```python
from build123d import *

# Parameters (mm, degrees)
SKETCH_1_R           = 7
EXTRUDE_1_DEPTH      = 30
SKETCH_2_W           = 5
SKETCH_2_H           = 5
EXTRUDE_2_DEPTH      = 0.1
EXTRUDE_2_DEPTH_BACK = 20
SKETCH_3_R           = 9
EXTRUDE_3_DEPTH      = 4
SKETCH_4_R           = 80
SKETCH_4_R_2         = 52
EXTRUDE_4_DEPTH      = 10
SKETCH_5_R           = 53
EXTRUDE_5_DEPTH      = 26
SKETCH_7_R           = 55
SKETCH_7_R_2         = 52
EXTRUDE_6_DEPTH      = 7.5
CHAMFER_1_SIZE       = 0.5
SKETCH_8_R           = 5
CUT_EXTRUDE_1_DEPTH  = 31
SKETCH_10_R          = 56
EXTRUDE_7_DEPTH      = 110
SKETCH_11_R          = 56.5
EXTRUDE_8_DEPTH      = 57
CHAMFER_2_SIZE       = 19
EXTRUDE_9_DEPTH      = 100
CUT_EXTRUDE_2_REACH  = 145
SKETCH_13_R          = 3.5
SKETCH_14_W          = 50
SKETCH_14_H          = 50
EXTRUDE_10_DEPTH     = 91
SKETCH_15_R          = 15
EXTRUDE_11_DEPTH     = 58
CHAMFER_3_SIZE       = 1
SKETCH_17_R          = 4
SKETCH_18_R          = 7
EXTRUDE_12_DEPTH     = 4
EXTRUDE_13_DEPTH     = 7
SKETCH_20_R          = 4
CUT_EXTRUDE_3_DEPTH  = 7


with BuildPart() as part:
    # Sketch 1 → Extrude 1 (new body)
    with BuildSketch(Plane.XY):
        Circle(SKETCH_1_R)
    extrude(amount=EXTRUDE_1_DEPTH)

    # Sketch 2 → Extrude 2 (add, two sides)
    with BuildSketch(Plane(origin=(0, 0, 0), x_dir=(-1, 0, 0), z_dir=(0, 0, -1))) as extrude_2_sk:
        with Locations((0, 6.5)):
            Rectangle(SKETCH_2_W, SKETCH_2_H)
    extrude(amount=EXTRUDE_2_DEPTH)
    extrude(extrude_2_sk.sketch, amount=-EXTRUDE_2_DEPTH_BACK)

    # Sketch 3 → Extrude 3 (add)
    with BuildSketch(Plane.XY.offset(30)):
        Circle(SKETCH_3_R)
    extrude(amount=EXTRUDE_3_DEPTH)



with BuildPart() as body_2:
    # Sketch 4 → Extrude 4 (new body)
    with BuildSketch(Plane(origin=(0, 0, 30), x_dir=(-1, 0, 0), z_dir=(0, 0, -1))):
        Circle(SKETCH_4_R)
        Circle(SKETCH_4_R_2, mode=Mode.SUBTRACT)
    extrude(amount=-EXTRUDE_4_DEPTH)


with BuildPart() as part_1:
    add(part.part)

    add(body_2.part)  # Extrude 5 merges body 2
    # Sketch 5 → Extrude 5 (add)
    with BuildSketch(Plane.XY.offset(34)):
        with Locations(Location((0, 0, 0), (0, 0, 180))):  # turned: the seam where the file's is
            Circle(SKETCH_5_R)
    extrude(amount=EXTRUDE_5_DEPTH)

    # Sketch 7 → Extrude 6 (add)
    with BuildSketch(Plane(origin=(0, 0, 34), x_dir=(-1, 0, 0), z_dir=(0, 0, -1))):
        Circle(SKETCH_7_R)
        Circle(SKETCH_7_R_2, mode=Mode.SUBTRACT)
    extrude(amount=EXTRUDE_6_DEPTH)

    # Chamfer 1
    chamfer_1_edges = [part_1.edges().sort_by_distance(p)[0] for p in [
        (55, 0, 26.5),
        (-3.968626967, -5.766281297, 0),
    ]]
    chamfer(chamfer_1_edges, length=CHAMFER_1_SIZE)

    # Sketch 8 → Cut-Extrude 1 (cut, through all)
    with BuildSketch(Plane(origin=(0, 0, 30), x_dir=(-1, 0, 0), z_dir=(0, 0, -1))):
        with Locations((-24.874423104, 60.052169613)):
            Circle(SKETCH_8_R)
        with Locations((24.874423104, 60.052169613)):
            Circle(SKETCH_8_R)
        with Locations((60.052169613, 24.874423104)):
            Circle(SKETCH_8_R)
        with Locations((60.052169613, -24.874423104)):
            Circle(SKETCH_8_R)
        with Locations((24.874423104, -60.052169613)):
            Circle(SKETCH_8_R)
        with Locations((-24.874423104, -60.052169613)):
            Circle(SKETCH_8_R)
        with Locations((-60.052169613, -24.874423104)):
            Circle(SKETCH_8_R)
        with Locations((-60.052169613, 24.874423104)):
            Circle(SKETCH_8_R)
    extrude(amount=-CUT_EXTRUDE_1_DEPTH, mode=Mode.SUBTRACT)

    # Sketch 10 → Extrude 7 (add)
    with BuildSketch(Plane.XY.offset(60)):
        Circle(SKETCH_10_R)
    extrude(amount=EXTRUDE_7_DEPTH)

    # Sketch 11 → Extrude 8 (add)
    with BuildSketch(Plane.XY.offset(170)):
        Circle(SKETCH_11_R)
    extrude(amount=EXTRUDE_8_DEPTH)

    # Chamfer 2
    chamfer_2_edges = [part_1.edges().sort_by_distance(p)[0] for p in [
        (-56.5, 0, 227),
    ]]
    chamfer(chamfer_2_edges, length=CHAMFER_2_SIZE)

    # Sketch 12 → Extrude 9 (add)
    with BuildSketch(Plane(origin=(0, 0, 60), x_dir=(-1, 0, 0), z_dir=(0, 0, -1))):
        Polygon((-60, -56), (-40.169137476, -56), (-29.800227926, -45.631090449), (-23.461287878, -49.191645338), (-37.26964254, -63), (-60, -63), align=None)
        Polygon((41.115933076, -56), (60, -56), (60, -63), (38.21643814, -63), (24.472073526, -49.255635387), (30.369884473, -45.253951397), align=None)
    extrude(amount=-EXTRUDE_9_DEPTH)

    # Sketch 13 → Cut-Extrude 2 (cut, up to next)
    with BuildSketch(Plane.XZ.offset(63), mode=Mode.PRIVATE) as cut_extrude_2_sk1:
        with Locations((-50, 70)):
            Circle(SKETCH_13_R)
    cut_extrude_2_tool1 = extrude(cut_extrude_2_sk1.sketch, amount=-CUT_EXTRUDE_2_REACH, mode=Mode.PRIVATE) & part_1.part
    add(cut_extrude_2_tool1.solids().sort_by_distance((-50, -63, 70))[0], mode=Mode.SUBTRACT)
    # Sketch 13 → Cut-Extrude 2 (cut, up to next)
    with BuildSketch(Plane.XZ.offset(63), mode=Mode.PRIVATE) as cut_extrude_2_sk2:
        with Locations((50, 70)):
            Circle(SKETCH_13_R)
    cut_extrude_2_tool2 = extrude(cut_extrude_2_sk2.sketch, amount=-CUT_EXTRUDE_2_REACH, mode=Mode.PRIVATE) & part_1.part
    add(cut_extrude_2_tool2.solids().sort_by_distance((50, -63, 70))[0], mode=Mode.SUBTRACT)
    # Sketch 13 → Cut-Extrude 2 (cut, up to next)
    with BuildSketch(Plane.XZ.offset(63), mode=Mode.PRIVATE) as cut_extrude_2_sk3:
        with Locations((-50, 150)):
            Circle(SKETCH_13_R)
    cut_extrude_2_tool3 = extrude(cut_extrude_2_sk3.sketch, amount=-CUT_EXTRUDE_2_REACH, mode=Mode.PRIVATE) & part_1.part
    add(cut_extrude_2_tool3.solids().sort_by_distance((-50, -63, 150))[0], mode=Mode.SUBTRACT)
    # Sketch 13 → Cut-Extrude 2 (cut, up to next)
    with BuildSketch(Plane.XZ.offset(63), mode=Mode.PRIVATE) as cut_extrude_2_sk4:
        with Locations((50, 150)):
            Circle(SKETCH_13_R)
    cut_extrude_2_tool4 = extrude(cut_extrude_2_sk4.sketch, amount=-CUT_EXTRUDE_2_REACH, mode=Mode.PRIVATE) & part_1.part
    add(cut_extrude_2_tool4.solids().sort_by_distance((50, -63, 150))[0], mode=Mode.SUBTRACT)

    # Sketch 14 → Extrude 10 (add)
    with BuildSketch(Plane(origin=(0, 0, 0), x_dir=(1, 0, 0), z_dir=(0, 1, 0))):
        with Locations((0, -86)):
            Rectangle(SKETCH_14_W, SKETCH_14_H)
    extrude(amount=EXTRUDE_10_DEPTH)

    # Sketch 15 → Extrude 11 (add)
    with BuildSketch(Plane(origin=(0, 0, 0), x_dir=(1, 0, 0), z_dir=(0, 1, 0))):
        with Locations(Location((0, -135, 0), (0, 0, 90))):  # turned: the seam where the file's is
            Circle(SKETCH_15_R)
    extrude(amount=EXTRUDE_11_DEPTH)

    # Chamfer 3
    chamfer_3_edges = [part_1.edges().sort_by_distance(p)[0] for p in [
        (0, 58, 150),
    ]]
    chamfer(chamfer_3_edges, length=CHAMFER_3_SIZE)

    # Sweep 1: sweep along a path in Sketch 16
    with BuildLine(Plane.XY.offset(135)) as sweep_1_path:
        CenterArc((0, 71), 13, 0, 360)
    # Sketch 17 → Sweep 1 (sweep)
    with BuildSketch(Plane(origin=(0, 0, 0), x_dir=(0, 0, -1), z_dir=(1, 0, 0))):
        with Locations((-135, 84)):
            Circle(SKETCH_17_R)
    sweep(path=sweep_1_path.line)

    # Sketch 18 → Extrude 12 (add)
    with BuildSketch(Plane.ZY.offset(25)):
        with Locations(Location((86, 69, 0), (0, 0, 180))):  # turned: the seam where the file's is
            Circle(SKETCH_18_R)
    extrude(amount=EXTRUDE_12_DEPTH)

    # Sketch 19 → Extrude 13 (add)
    with BuildSketch(Plane.ZY.offset(29)):
        Polygon((86, 78.814954576), (77.5, 73.907477288), (77.5, 64.092522712), (86, 59.185045424), (94.5, 64.092522712), (94.5, 73.907477288), align=None)
    extrude(amount=EXTRUDE_13_DEPTH)

    # Sketch 20 → Cut-Extrude 3 (cut)
    with BuildSketch(Plane.ZY.offset(36)):
        with Locations((86, 69)):
            Circle(SKETCH_20_R)
    extrude(amount=-CUT_EXTRUDE_3_DEPTH, mode=Mode.SUBTRACT)


solid = part_1.part
```
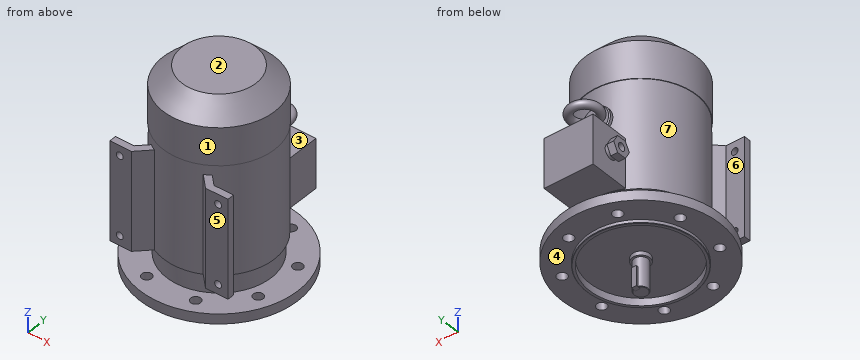
Here's how the part is built. I have some questions about the finished solid (model axes, mm). Face numbers are marked on the shaded views. A direction names the side the tool comes from. Coordinates: 2 decimals unless noted, no trailing zeros. Order: outer loops, then holes, each group sorted by start corner. A loop starts at its lowest first (then second) coordinate and runs counter-clockwise, first axis right, second up.
1) We'd pull the mould along Z, two halves only. Please class the marked faces 1, 2 and 3: +Z half, -Z half, draft (parallel to the pull), parting line (faces both ways), or undercut.
2) I need wall thicknesses on line 1 (Z direction, x = -50, y = -61); line 2 (X direction, y = 27, z = 37); line 3 (X direction, y = -58, z = 150). Which ranges of each line are inside material? Lowest first, please.
3) Which directions (+Z, -Z, +X, -X, +Y, -Y) give clear straight access to the entire face, cutting with the end or side of a thin tool? Please do the marked faces 4, 5, 6 and 7.
4) Imagine slicing it at B-B on z = 16.5. List the corners of the cut face in (x, y) for me.
5) Will these pins go through, and if not, where does the flat tip stop? pin 1 (12.5 mm diameter, centred on x = -9.5, y = 77.5, fed in from -Z); pin 2 (1 mm diameter, centred on y = 30, z = 61, fed in from +X); pin 3 (6 mm diameter, centred on x = -11, z = 133.5, fed in from +Y).
6) Imagine slicing it at A-A on z = 70. List the corners of the cut face in (x, y) for me, and give its area (3 significant figures).
Response values:
1. face 1: draft
1. face 2: +Z half
1. face 3: undercut
2. line 1: z = 30 to 40, 60 to 66.5, 73.5 to 146.5, 153.5 to 160
2. line 2: x = -75.31 to -64.58, -55.53 to 55.53, 64.58 to 75.31
2. line 3: x = -60 to -53.5, -46.5 to -33.22, 32.27 to 46.5, 53.5 to 60
3. face 4: -Z
3. face 5: +Z, +X, -X, -Y
3. face 6: +Z, -X
3. face 7: none
4. outline: (-2.5, 6.54) arc R7 ccw (long way) to (2.5, 6.54) - (2.5, 9) - (-2.5, 9) - close
5. pin 1: stops at z = 30
5. pin 2: stops at x = 47.6
5. pin 3: stops at y = 85.87
6. outline: (-60, -63) - (-53.5, -63) - (-53.5, -56) - (-60, -56) - close; (-46.5, -63) - (-38.22, -63) - (-25.22, -50) arc R56 ccw to (24.58, -50.31) - (37.27, -63) - (46.5, -63) - (46.5, -56) - (40.17, -56) - (30.88, -46.71) arc R56 ccw to (25, 50.11) - (25, 91) - (-25, 91) - (-25, 50.11) arc R56 ccw to (-31.45, -46.33) - (-41.12, -56) - (-46.5, -56) - close; (53.5, -63) - (60, -63) - (60, -56) - (53.5, -56) - close
6. area: 12,100 mm2
